Geometry: final body of the model. Coordinates: model frame, mm. Round coordinates to 2 decimals unless told otherwise and drop trailing zeros. Loops run counter-clockwise (first coordinate to the right, second up) from the corner with the lowest first, then second, coordinate; pieces in that order, holes last. Notation, with made-up numbers: (39.25, 7) - (48.25, 7) arc R31 ccw to (48.25, 44) - close; hole circle Ø8 at (-9, 0.5). An arc over 180 degrees is marked (long way). Answer as a JSON object with one key per item and string values. Group by question number.
Item 1: Section C-C (z = 2). Count the separate pieces of the cut face and the enclosed holes in it, plus the area to 3 significant figures.
Item 2: Section A-A (x = 36.5). Return the cut outline in (y, z).
Item 3: Line query: line 1 (Y direction, x = 68, z = 1.2); line 2 (Y direction, x = 40.5, z = 1.25); line 3 (Y direction, x = -12, z = 1.2). Output: solid intervals per line, ascending.
Item 4: Section B-B (y = -13.5). Return the cut outline in (x, z).
Item 5: Section D-D (x = 80.5). Return the cut outline in (y, z), plus the area to 3 significant figures.
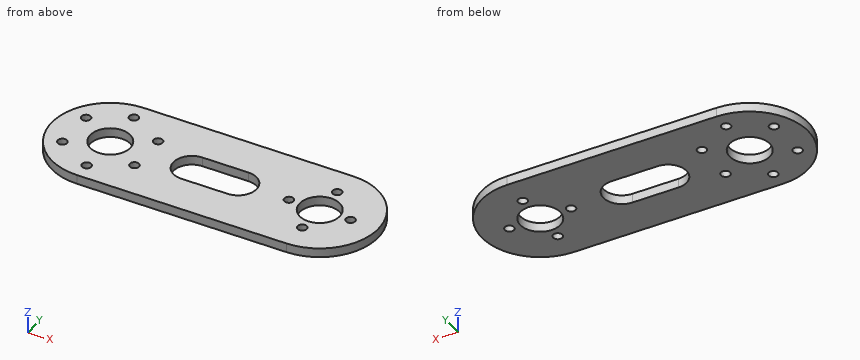
```python
from build123d import *

# Parameters (mm, degrees)
SKETCH_1_R          = 19
SKETCH_1_R_2        = 1.5
SKETCH_1_R_3        = 6.5
EXTRUDE_1_DEPTH     = 3
SKETCH_2_R          = 6.5
CUT_EXTRUDE_1_DEPTH = 90.101066211


with BuildPart() as part:
    # 草图1 → 凸台-拉伸1 (new body)
    # profile 1 of 3: a face of its own
    with BuildSketch(Plane.XY):
        Circle(SKETCH_1_R)
        with Locations((0, 13.5)):
            Circle(SKETCH_1_R_2, mode=Mode.SUBTRACT)
        with Locations((11.691342951, 6.75)):
            Circle(SKETCH_1_R_2, mode=Mode.SUBTRACT)
        with Locations((11.691342951, -6.75)):
            Circle(SKETCH_1_R_2, mode=Mode.SUBTRACT)
        with Locations((0, -13.5)):
            Circle(SKETCH_1_R_2, mode=Mode.SUBTRACT)
        with Locations((-11.691342951, -6.75)):
            Circle(SKETCH_1_R_2, mode=Mode.SUBTRACT)
        with Locations((-11.691342951, 6.75)):
            Circle(SKETCH_1_R_2, mode=Mode.SUBTRACT)
        Circle(SKETCH_1_R_3, mode=Mode.SUBTRACT)
    # profile 2 of 3: a face of its own
    with BuildSketch(Plane.XY):
        with BuildLine():
            Line((68, 19), (0, 19))
            ThreePointArc((0, 19), (13.435028843, 13.435028843), (19, 0))
            ThreePointArc((19, 0), (13.435028843, -13.435028843), (0, -19))
            Line((0, -19), (68, -19))
            ThreePointArc((68, -19), (49, 0), (68, 19))
        make_face()
    # profile 3 of 3: a face of its own
    with BuildSketch(Plane.XY):
        with Locations((68, 0)):
            Circle(SKETCH_1_R)
        with Locations((68, 0)):
            Circle(SKETCH_1_R_3, mode=Mode.SUBTRACT)
        with Locations((68, 10)):
            Circle(SKETCH_1_R_2, mode=Mode.SUBTRACT)
        with Locations((78, 0)):
            Circle(SKETCH_1_R_2, mode=Mode.SUBTRACT)
        with Locations((68, -10)):
            Circle(SKETCH_1_R_2, mode=Mode.SUBTRACT)
        with Locations((58, 0)):
            Circle(SKETCH_1_R_2, mode=Mode.SUBTRACT)
    extrude(amount=EXTRUDE_1_DEPTH)

    # 草图2 → 切除-拉伸1 (cut, through all)
    with BuildSketch(Plane.XY.offset(3)):
        with Locations((68, 0)):
            Circle(SKETCH_2_R)
        with BuildLine():
            Line((26.5, 6), (41.5, 6))
            ThreePointArc((41.5, 6), (47.5, 0), (41.5, -6))
            Line((41.5, -6), (26.5, -6))
            ThreePointArc((26.5, -6), (20.5, 0), (26.5, 6))
        make_face()
    extrude(amount=-CUT_EXTRUDE_1_DEPTH, mode=Mode.SUBTRACT)


solid = part.part
```
Values:
{
 "1": {"separate pieces": "1", "enclosed holes": "13", "area": "3,090 mm^2"},
 "2": {"outline": "(-19, 0) - (-6, 0) - (-6, 3) - (-19, 3) - close; (6, 0) - (19, 0) - (19, 3) - (6, 3) - close"},
 "3": {"line 1": "y = -19 to -11.5, -8.5 to -6.5, 6.5 to 8.5, 11.5 to 19", "line 2": "y = -19 to -6, 6 to 19", "line 3": "y = -14.73 to -8.22, -5.28 to 5.28, 8.22 to 14.73"},
 "4": {"outline": "(-13.37, 0) - (-1.5, 0) - (-1.5, 3) - (-13.37, 3) - close; (1.5, 0) - (81.37, 0) - (81.37, 3) - (1.5, 3) - close"},
 "5": {"outline": "(-14.31, 0) - (14.31, 0) - (14.31, 3) - (-14.31, 3) - close", "area": "85.9 mm^2"}
}
